Verification items for the finished model (mm, model axes). A direction names the side the tool comes from. Round coordinates to 2 decimals unless told otherwise and drop trailing zeros. Write each loop counter-clockwise with the first axis right and the second up, starting at its lowest first coordinate (ties: lowest second). Pieces come first, ordered by that corner, then holes. Notation, with made-up numbers: (13.25, 0.25) - (30.25, 0.25) arc R28 cw to (30.25, 35.25) - close; hole circle Ø5 at (-29.75, 49.25). An arc over 180 degrees is marked (long way). Answer as a JSON object with one key per item and string values.
```python
from build123d import *

# Parameters (mm, degrees)
SKETCH_1_R          = 10
EXTRUDE_1_DEPTH     = 94
CUT_EXTRUDE_1_DEPTH = 30
SKETCH_3_R          = 1.5
CUT_EXTRUDE_2_DEPTH = 95
SKETCH_4_R          = 25
SKETCH_4_R_2        = 1.5
EXTRUDE_2_DEPTH     = 4
SKETCH_5_R          = 1.5
CUT_EXTRUDE_5_DEPTH = 4


with BuildPart() as part:
    # 草图1 → 凸台-拉伸1 (new body)
    with BuildSketch(Plane.XY):
        Circle(SKETCH_1_R)
    extrude(amount=EXTRUDE_1_DEPTH)

    # 草图2 → 切除-拉伸1 (cut)
    with BuildSketch(Plane.XY.offset(94)):
        with BuildLine():
            Line((-2.5, 6.538348415), (-2.5, 9.2))
            Line((-2.5, 9.2), (2.5, 9.2))
            Line((2.5, 9.2), (2.5, 6.538348415))
            ThreePointArc((2.5, 6.538348415), (0, -7), (-2.5, 6.538348415))
        make_face()
    extrude(amount=-CUT_EXTRUDE_1_DEPTH, mode=Mode.SUBTRACT)

    # 草图3 → 切除-拉伸2 (cut, through all)
    with BuildSketch(Plane(origin=(0, 0, 0), x_dir=(-1, 0, 0), z_dir=(0, 0, -1))):
        Circle(SKETCH_3_R)
    extrude(amount=-CUT_EXTRUDE_2_DEPTH, mode=Mode.SUBTRACT)

    # 草图4 → 凸台-拉伸2 (add)
    with BuildSketch(Plane(origin=(0, 0, 0), x_dir=(-1, 0, 0), z_dir=(0, 0, -1))):
        Circle(SKETCH_4_R)
        Circle(SKETCH_4_R_2, mode=Mode.SUBTRACT)
    extrude(amount=EXTRUDE_2_DEPTH)

    # 草图5 → 切除-拉伸5 (cut)
    with BuildSketch(Plane(origin=(0, 0, -4), x_dir=(-1, 0, 0), z_dir=(0, 0, -1))):
        with Locations((0, 15)):
            Circle(SKETCH_5_R)
        with Locations((12.990381057, 7.5)):
            Circle(SKETCH_5_R)
        with Locations((12.990381057, -7.5)):
            Circle(SKETCH_5_R)
        with Locations((0, -15)):
            Circle(SKETCH_5_R)
        with Locations((-12.990381057, -7.5)):
            Circle(SKETCH_5_R)
        with Locations((-12.990381057, 7.5)):
            Circle(SKETCH_5_R)
    extrude(amount=-CUT_EXTRUDE_5_DEPTH, mode=Mode.SUBTRACT)


solid = part.part
```
Q1. Release check for a two-part mould opening along X. For faces 3 (the flat face through (-7, -2, 94)), 4 (the cylindrical face through (-2.17, -9.76, 46.34)), 5 (the flat face through (0, 9.2, 79)) record: released by +X, released by -X, zero draft, split by the parting line, or undercut.
Geometry check:
{"face 3": "zero draft", "face 4": "split by the parting line", "face 5": "undercut"}
Q2. Section check D-D, the plane z = 56.5. Record the cut outline in (x, y).
Geometry check:
{"outline": "circle Ø20 at (0, 0); hole circle Ø3 at (0, 0)"}
Q3. Material ranges on line 1 along Y through (x, z) = (-0.5, 70); line 2 along Z through (x, y) = (2.5, 22.5); line 3 along Y through (x, z) = (-4, 79.5), recorded low to high. Write a range as [from, to].
Geometry check:
{"line 1": "y = [-9.99, -6.98], [9.2, 9.99]", "line 2": "z = [-4, 0]", "line 3": "y = [-9.17, -5.74], [5.74, 9.17]"}
Q4. Section check B-B, the plane x = 0. Record the cut outline in (y, z).
Geometry check:
{"outline": "(-25, -4) - (-16.5, -4) - (-16.5, 0) - (-25, 0) - close; (-13.5, -4) - (-1.5, -4) - (-1.5, 64) - (-7, 64) - (-7, 94) - (-10, 94) - (-10, 0) - (-13.5, 0) - close; (1.5, -4) - (13.5, -4) - (13.5, 0) - (10, 0) - (10, 94) - (9.2, 94) - (9.2, 64) - (1.5, 64) - close; (16.5, -4) - (25, -4) - (25, 0) - (16.5, 0) - close"}
Q5. Section check A-A, the plane y = -15. Record the cut outline in (x, z).
Geometry check:
{"outline": "(-20, -4) - (-1.5, -4) - (-1.5, 0) - (-20, 0) - close; (1.5, -4) - (20, -4) - (20, 0) - (1.5, 0) - close"}
Q6. Set-up check for faces 1 (the cylindrical face through (0.325, -16.464, -2.028)), 2 (the flat face through (-1.5, 1.2, 64)): record each of +Z, -Z, +X, -X, +Y, -Y from which the full face is reachable in a straight line by a thin tool's end or side.
Geometry check:
{"face 1": "+Z, -Z", "face 2": "+Z"}
Q7. Section check C-C, the plane y = 2.5. Record the cut outline in (x, z).
Geometry check:
{"outline": "(-24.87, -4) - (24.87, -4) - (24.87, 0) - (9.68, 0) - (9.68, 94) - (6.54, 94) - (6.54, 64) - (-6.54, 64) - (-6.54, 94) - (-9.68, 94) - (-9.68, 0) - (-24.87, 0) - close"}
Q8. Gauge pin test, flat ends, axial feed: P1, Ø5, axis at x = 4, z = 44.5, coming from the -Y side; P2, Ø10, axis at x = 13.5, z = 43, coming from the +Y side; P3, Ø12, axis at x = 13.5, y = 14.5, coming from the +Z side. Record the tip position at first contact, or that the pin passes through.
Geometry check:
{"P1": "stops at y = -9.89", "P2": "stops at y = 5.27", "P3": "stops at z = 0"}
